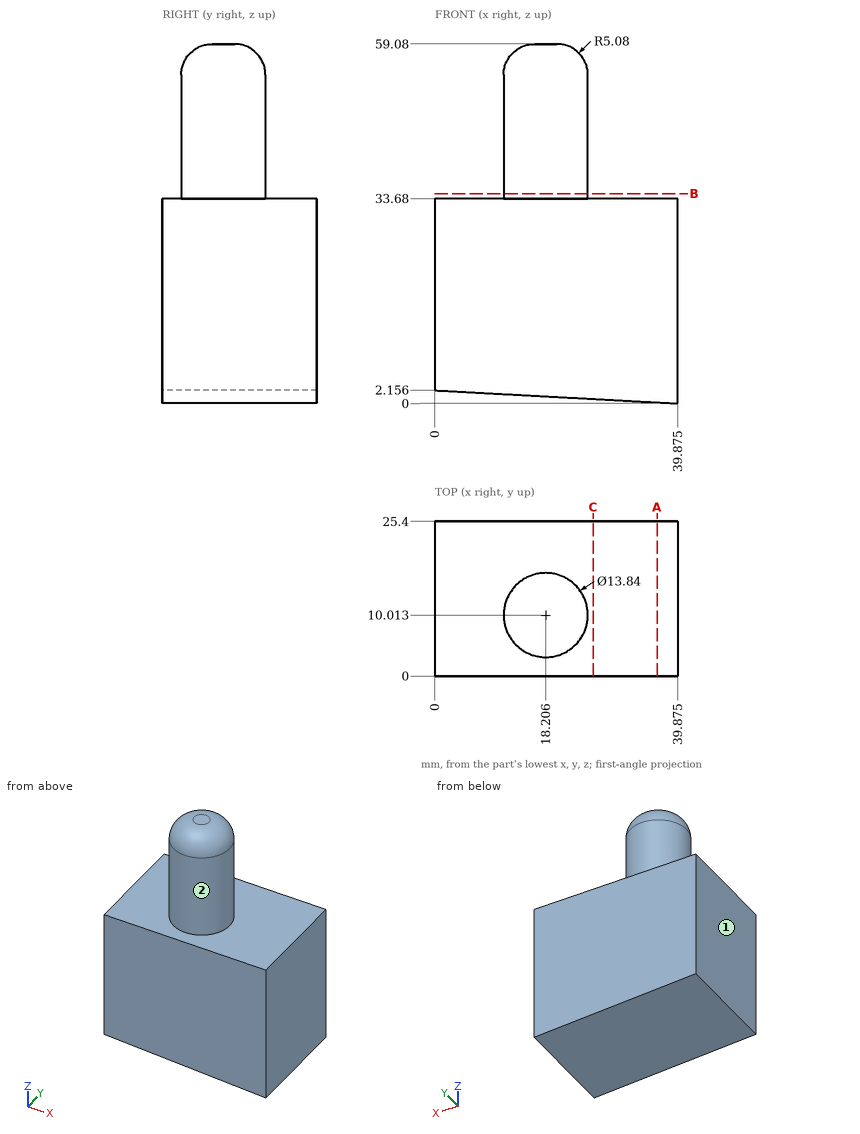
Geometry: see drawing. Coordinates: mm, zero at the bounding-box minimum. A direction names the side the tool comes from. Give positions to 0.01 mm unless a question says otherwise; leave off trailing zeros. Order: outer loops, then holes, each group sorted by start corner. A loop starts at its lowest first (then second) coordinate and runs counter-clockwise, first axis right, second up. Notation, with made-up numbers: (74, 5.25) - (101, 5.25) arc R25 cw to (101, 34.25) - close; hole circle Ø6 at (25.5, 15). An arc over 180 degrees is marked (long way). One line per item, written item: value.
1. Line query: probe 1 along Z at (x, y) = (34, 15.75); probe 2 along X at (y, z) = (14, 50); probe 3 along X at (y, z) = (4.75, 42) (1 decimal). Output: solid intervals per line, ascending.
Determined:
probe 1: 0.32 to 33.68
probe 2: 12.55 to 23.86
probe 3: 13.7 to 22.7
2. Cut plane C-C, the plane x = 26. Output: boundary loops of the cut face in (y, z).
Determined:
outline: (0, 0.75) - (25.4, 0.75) - (25.4, 33.68) - (0, 33.68) - close
3. Pin query (flat end, axial travel): pin 1 Ø4 at (y, z) = (12.5, 51) entering from -X; pin 2 Ø8 at (x, y) = (16.5, 15) entering from -Z; pin 3 Ø5 at (x, y) = (5.5, 17.5) entering from -Z. Return the tip coordinate at first contact, or that it passes through.
Determined:
pin 1: x = 11.3
pin 2: z = 1.05
pin 3: z = 1.72
4. Cut plane A-A, the plane x = 36.5. Output: boundary loops of the cut face in (y, z).
Determined:
outline: (0, 0.18) - (25.4, 0.18) - (25.4, 33.68) - (0, 33.68) - close
5. Reachability of the marked faces 1 and 2 from +Z, -Z, +X, -X, +Y, -Y: full face, straight path, thin tool, end or side. Return the list, or none.
Determined:
face 1: +Z, -Z, -X, +Y, -Y
face 2: +Z
6. Cut plane B-B, the plane z = 34.5. Output: boundary loops of the cut face in (x, y), and give its area (3 significant figures).
Determined:
outline: circle Ø13.84 at (18.21, 10.01)
area: 150 mm2
